from build123d import *

# Parameters (mm, degrees)
SKETCH1_R                = 3.2639
SKETCH1_R_2              = 12.7
BOSS_EXTRUDE1_DEPTH      = 3.175
SKETCH2_R                = 12.7
SKETCH2_R_2              = 7.9375
BOSS_EXTRUDE2_DEPTH      = 34.925
BOSS_EXTRUDE2_DEPTH_BACK = 3.175
SKETCH4_W                = 4.953
SKETCH4_H                = 19.558
BOSS_EXTRUDE3_DEPTH      = 3.175
SKETCH5_W                = 9.525
SKETCH5_H                = 3.302
CUT_EXTRUDE1_DEPTH       = 39.1


with BuildPart() as part:
    # Sketch1 → Boss-Extrude1 (new body)
    with BuildSketch(Plane(origin=(0, 0, 0), x_dir=(0, 0, -1), z_dir=(1, 0, 0))):
        with BuildLine():
            Line((106.143178695, 13.781217887), (47.625, 26.9875))
            Line((47.625, 26.9875), (-47.625, 26.9875))
            Line((-47.625, 26.9875), (-47.625, -26.9875))
            Line((-47.625, -26.9875), (101.6, -26.9875))
            ThreePointArc((101.6, -26.9875), (122.110538942, -8.635650576), (106.143178695, 13.781217887))
        make_face()
        with Locations((38.1, 17.4625)):
            Circle(SKETCH1_R, mode=Mode.SUBTRACT)
        with Locations((38.1, -17.4625)):
            Circle(SKETCH1_R, mode=Mode.SUBTRACT)
        with Locations((-38.1, -17.4625)):
            Circle(SKETCH1_R, mode=Mode.SUBTRACT)
        with Locations((-38.1, 17.4625)):
            Circle(SKETCH1_R, mode=Mode.SUBTRACT)
        with Locations((101.6, -6.35)):
            Circle(SKETCH1_R_2, mode=Mode.SUBTRACT)
    extrude(amount=BOSS_EXTRUDE1_DEPTH)

    # Sketch2 → Boss-Extrude2 (add, two sides)
    with BuildSketch(Plane.ZY) as boss_extrude2_sk:
        with Locations((-101.6, -6.35)):
            Circle(SKETCH2_R)
        with Locations((-101.6, -6.35)):
            Circle(SKETCH2_R_2, mode=Mode.SUBTRACT)
    extrude(amount=BOSS_EXTRUDE2_DEPTH)
    extrude(boss_extrude2_sk.sketch, amount=-BOSS_EXTRUDE2_DEPTH_BACK)

    # Sketch4 → Boss-Extrude3 (add)
    with BuildSketch(Plane(origin=(3.175, 0, 0), x_dir=(0, 0, -1), z_dir=(1, 0, 0))):
        with BuildLine():
            Line((-47.625, 26.9875), (-60.325, 26.9875))
            ThreePointArc((-60.325, 26.9875), (-69.305256121, 23.267756121), (-73.025, 14.2875))
            Line((-73.025, 14.2875), (-73.025, -14.2875))
            ThreePointArc((-73.025, -14.2875), (-69.305256121, -23.267756121), (-60.325, -26.9875))
            Line((-60.325, -26.9875), (-47.625, -26.9875))
            Line((-47.625, -26.9875), (-47.625, 26.9875))
        make_face()
        with Locations((-58.1025, 0)):
            Rectangle(SKETCH4_W, SKETCH4_H, mode=Mode.SUBTRACT)
    extrude(amount=-BOSS_EXTRUDE3_DEPTH)

    # Sketch5 → Cut-Extrude1 (cut, through all)
    with BuildSketch(Plane(origin=(3.175, 0, 0), x_dir=(0, 0, -1), z_dir=(1, 0, 0))):
        with Locations((20.6375, -6.2865)):
            Rectangle(SKETCH5_W, SKETCH5_H)
        with Locations((-7.9375, -6.2865)):
            Rectangle(SKETCH5_W, SKETCH5_H)
    extrude(amount=-CUT_EXTRUDE1_DEPTH, mode=Mode.SUBTRACT)


solid = part.part
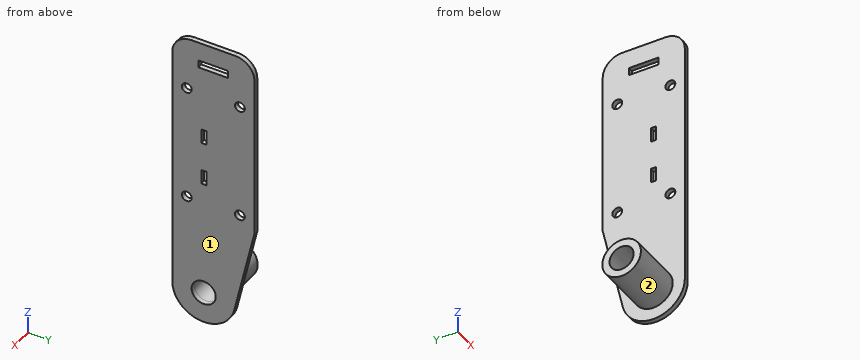
The model under review builds one solid part; all positions refer to its coordinate system, in mm. Face numbers are marked on the shaded views. A direction names the side the tool comes from. Round coordinates to 2 decimals unless told otherwise and drop trailing zeros. Loops run counter-clockwise (first coordinate to the right, second up) from the corner with the lowest first, then second, coordinate; pieces in that order, holes last. Notation, with made-up numbers: (25, 52.25) -> (82, 52.25) arc R19 cw to (82, 59.25) -> close; hole circle Ø4 at (72.25, 8.5). An arc over 180 degrees is marked (long way). One line per question, with ' | ' between items. Start each with the question number.
Item 1: For pin 1 (12 mm diameter, centred on y = 12.5, z = 23.5, fed in from -X); pin 2 (3.5 mm diameter, centred on x = 2, y = 1, fed in from -Z); pin 3 (2.5 mm diameter, centred on x = 1, y = -5.5, fed in from -Z); pin 4 (2 mm diameter, centred on x = -10, y = 0.5, fed in from +Z), all flat-tipped, find the tip position at first contact; note any pin that passes through.
Item 2: Machinability: for the marked faces 1 and 2, which of the approach directions +Z, -Z, +X, -X, +Y, -Y give a long, thin tool a straight path to every point of the face, cutting with its end or side? Answer none if there is none.
Item 3: Add section C-C, the plane z = -98. Write out the cut boundary in (x, y) (1 decimal), then the cut area to 3 significant figures.
Item 4: Wall thickness on line 1 along Y through (x, z) = (1.7, -38.1); line 2 along Y through (x, z) = (-11, -101.6); line 3 along X through (y, z) = (14, 45.5) (3 decimals): over which ranges is each line inside the solid? List them lowest first. Write a range as [from, to].
Item 5: Add section D-D, the plane z = 44.5. Write out the cut boundary in (x, y) (1 decimal).
Item 6: Add section A-A, the plane z = -22. Write out the cut boundary in (x, y) (1 decimal).
Return value:
1) pin 1: stops at x = 0 | pin 2: stops at z = -121.46 | pin 3: stops at z = -122.24 | pin 4: stops at z = -90.33
2) face 1: +Z, -Z, +X, +Y, -Y | face 2: -X
3) outline: (-34.9, -18.5) -> (0, -18.5) -> (0, -27) -> (3.2, -27) -> (3.2, -13.4) -> (-34.9, -13.4) -> close; (-34.9, 0.7) -> (3.2, 0.7) -> (3.2, 15.6) -> (0, 15.6) -> (0, 5.8) -> (-34.9, 5.8) -> close | area: 447 mm2
4) line 1: y = [-26.99, -20.73], [-14.2, 14.2], [20.73, 26.99] | line 2: y = [-19.05, -14.29], [1.59, 6.35] | line 3: x = [0, 3.175]
5) outline: (0, -27) -> (3.2, -27) -> (3.2, 27) -> (0, 27) -> close
6) outline: (0, -27) -> (3.2, -27) -> (3.2, -7.9) -> (0, -7.9) -> close; (0, -4.6) -> (3.2, -4.6) -> (3.2, 27) -> (0, 27) -> close
